from build123d import *

# Parameters (mm, degrees)
F1_DEPTH = 50.8
F2_R     = 3.175
F3_DEPTH = 25.4


with BuildPart() as f1:
    # F0 (on Right) → F1 (new body)
    with BuildSketch(Plane.YZ):
        with BuildLine():
            ThreePointArc((12.7, 0), (11.770064, 2.245064), (9.525, 3.175))
            Line((9.525, 3.175), (-12.7, 3.175))
            ThreePointArc((-12.7, 3.175), (-14.945064, 4.104936), (-15.875, 6.35))
            Line((-15.875, 6.35), (-15.875, 6.919573))
            ThreePointArc((-15.875, 6.919573), (-20.851669, 12.382725), (-19.05, 5.21563))
            Line((-19.05, 5.21563), (-18.026482, 5.21563))
            ThreePointArc((-18.026482, 5.21563), (-17.627686, 5.050443), (-17.4625, 4.651648))
            Line((-17.4625, 4.651648), (-17.4625, 0))
            ThreePointArc((-17.4625, 0), (-16.532564, -2.245064), (-14.2875, -3.175))
            Line((-14.2875, -3.175), (-12.7, -3.175))
            Line((-12.7, -3.175), (9.525, -3.175))
            ThreePointArc((9.525, -3.175), (11.770064, -2.245064), (12.7, 0))
        make_face()
        with BuildLine():
            ThreePointArc((-15.5575, 9.02563), (-16.58043, 6.556059), (-19.05, 5.53313))
            ThreePointArc((-19.05, 5.53313), (-21.51957, 11.4952), (-15.5575, 9.02563))
        make_face(mode=Mode.SUBTRACT)
    extrude(amount=F1_DEPTH)

    # F2 (on face) → F3 (cut)
    with BuildSketch(Plane.XY.offset(3.175)):
        with Locations((41.275, -7.62)):
            Circle(F2_R)
        with Locations((41.275, 4.445)):
            Circle(F2_R)
        with Locations((9.525, 4.445)):
            Circle(F2_R)
        with Locations((9.525, -7.62)):
            Circle(F2_R)
    extrude(amount=-F3_DEPTH, mode=Mode.SUBTRACT)


solid = f1.part
Source: CAD feature listing. Evaluate the final solid. Frame: model axes, mm. A direction names the side the tool comes from. Round coordinates to 2 decimals unless told otherwise and drop trailing zeros. Loops run counter-clockwise (first coordinate to the right, second up) from the corner with the lowest first, then second, coordinate; pieces in that order, holes last. Notation, with made-up numbers: M -39,26.25 L 12,26.25 A17 cw 12,49.25 Z; hole C 18.25,54.5 d5. An arc over 180 degrees is marked long. Return JSON: item names as keys, results as strings. Group by question number.
1. Reachability of faces 4 (the face through (25, -17.462, 2)), 5 (the face through (12.46, 3.23, 0.04)) from +Z, -Z, +X, -X, +Y, -Y: full face, straight path, thin tool, end or side. Return the list, or none.
2. Pin query (flat end, axial travel): pin 1 (6.5 mm diameter, centred on x = 24.5, y = -5.5, fed in from +Z) (3 decimals); pin 2 (3 mm diameter, centred on x = 42, z = 5.5, fed in from +Y) (3 decimals); pin 3 (4 mm diameter, centred on x = 9.525, y = -7.62, fed in from -Z); pin 4 (2 mm diameter, centred on x = 34.5, z = 10.5, fed in from -Y). Return the tip coordinate at first contact, or that it passes through.
3. Mould query, pull axis Y, two halves, no side actions, for faces 1 (the face through (25, -1, 3.175)), 2 (the face through (38.103, -7.48, 0.044)), 3 (the face through (25.04, -14.92, 4.08)). Classes: released by +Y, released by -Y, zero draft, split by the parting line, or undercut.
4. Section query D-D on z = 11. Output: boundary loops of the cut face in (x, y).
5. Section query A-A on y = -7.62. Output: boundary loops of the cut face in (x, z) (3 decimals), and give its area (3 significant figures).
6. Section query B-B on z = 8. Output: boundary loops of the cut face in (x, y).
7. Material intervals for line 1 along Y through (x, z) = (44, 9); line 2 along Y through (x, z) = (10, 0.75); line 3 along X through (y, z) = (-6, -1), sorted ascending. Write a range as from..to.
Checks:
{
 "1": {"face 4": "-Z, +X, -X, -Y", "face 5": "+Z, -Z"},
 "2": {"pin 1": "stops at z = 3.175", "pin 2": "stops at y = -14.835", "pin 3": "passes through", "pin 4": "stops at y = -22.83"},
 "3": {"face 1": "zero draft", "face 2": "undercut", "face 3": "released by +Y"},
 "4": {"outline": "M 0,-22.31 L 50.8,-22.31 L 50.8,-21.93 L 0,-21.93 Z; M 0,-16.17 L 50.8,-16.17 L 50.8,-15.79 L 0,-15.79 Z"},
 "5": {"outline": "M 0,-3.175 L 6.35,-3.175 L 6.35,3.175 L 0,3.175 Z; M 12.7,-3.175 L 38.1,-3.175 L 38.1,3.175 L 12.7,3.175 Z; M 44.45,-3.175 L 50.8,-3.175 L 50.8,3.175 L 44.45,3.175 Z", "area": "242 mm²"},
 "6": {"outline": "M 0,-22.72 L 50.8,-22.72 L 50.8,-22.39 L 0,-22.39 Z; M 0,-15.71 L 50.8,-15.71 L 50.8,-15.38 L 0,-15.38 Z"},
 "7": {"line 1": "y = -22.86..-22.54, -15.56..-15.24", "line 2": "y = -17.46..-10.76, -4.48..1.31, 7.58..12.61", "line 3": "x = 0..6.79, 12.26..38.54, 44.01..50.8"}
}
